Job drawing, mm, ordinate dimensions from the low corner. One solid piece. Give positions to 0.01 mm unless a question says otherwise; leave off trailing zeros. Order: outer loops, then holes, each group sorted by start corner. A loop starts at its lowest first (then second) coordinate and runs counter-clockwise, first axis right, second up.
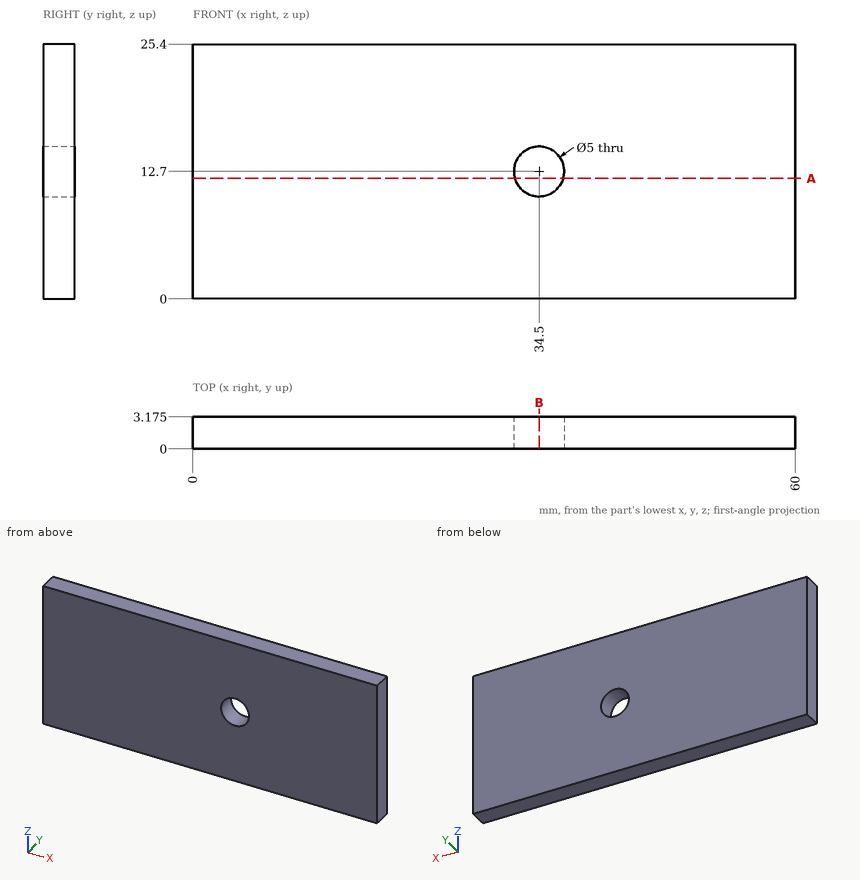
Item 1: Drill centre lines: probe 1 along X at (y, z) = (1.95, 12.7); probe 2 along Z at (x, y) = (34.5, 1.95); probe 3 along X at (y, z) = (0.95, 14.25). Where is each one in solid material? Low to high.
Item 2: Band-saw the part on A-A on z = 12. List the corners of the cut face in (x, y) (3 decimals).
Item 3: Band-saw the part on B-B on x = 34.5. List the corners of the cut face in (y, z) (3 decimals).
Working result:
1. probe 1: x = 0 to 32, 37 to 60
1. probe 2: z = 0 to 10.2, 15.2 to 25.4
1. probe 3: x = 0 to 32.54, 36.46 to 60
2. outline: (0, 0) - (32.1, 0) - (32.1, 3.175) - (0, 3.175) - close; (36.9, 0) - (60, 0) - (60, 3.175) - (36.9, 3.175) - close
3. outline: (0, 0) - (3.175, 0) - (3.175, 10.2) - (0, 10.2) - close; (0, 15.2) - (3.175, 15.2) - (3.175, 25.4) - (0, 25.4) - close
